Geometry check sheet. Reference: the model listing, model coordinates, mm. A direction names the side the tool comes from. Coordinates: 2 decimals unless noted, no trailing zeros. Write each loop counter-clockwise with the first axis right and the second up, starting at its lowest first coordinate (ties: lowest second). Pieces come first, ordered by that corner, then holes. Notation, with made-up numbers: M -35,3 L 16,3 A34 ccw 16,34 Z; hole C 82.5,70.5 d4. An arc over 180 degrees is marked long. Write each question's results on one line, items separated by ' | '.
```python
from build123d import *

# Parameters (mm, degrees)
REVOLVE1_ANGLE = 72


with BuildPart() as part:
    # Sketch1 → Revolve1 (revolve)
    with BuildSketch(Plane.XY):
        with BuildLine():
            ThreePointArc((-52.157480315, 97.330708661), (-49.814334564, 102.987562911), (-44.157480315, 105.330708661))
            Line((-44.157480315, 105.330708661), (6.842519685, 105.330708661))
            ThreePointArc((6.842519685, 105.330708661), (12.499373935, 102.987562911), (14.842519685, 97.330708661))
            Line((14.842519685, 97.330708661), (14.842519685, 70.330708661))
            Line((14.842519685, 70.330708661), (10.842519685, 70.330708661))
            Line((10.842519685, 70.330708661), (10.842519685, 97.330708661))
            ThreePointArc((10.842519685, 97.330708661), (9.67094681, 100.159135786), (6.842519685, 101.330708661))
            Line((6.842519685, 101.330708661), (-44.157480315, 101.330708661))
            ThreePointArc((-44.157480315, 101.330708661), (-46.98590744, 100.159135786), (-48.157480315, 97.330708661))
            Line((-48.157480315, 97.330708661), (-48.157480315, 70.330708661))
            Line((-48.157480315, 70.330708661), (-52.157480315, 70.330708661))
            Line((-52.157480315, 70.330708661), (-52.157480315, 97.330708661))
        make_face()
    revolve(axis=Axis((14.842519685, -1144.669291339, 0), (-1, 0, 0)), revolution_arc=REVOLVE1_ANGLE)


solid = part.part
```
Q1. Depth check by flat-ended pin: P1, Ø12, axis at x = 7, y = -155.5, coming from the +Z side; P2, Ø8, axis at x = -5, z = -196, coming from the -Y side; P3, Ø6, axis at x = 1.5, z = -266, coming from the +Y side. Enter the tip coordinate at first touch or a pass-through.
Geometry check:
P1: stops at z = -699.02 | P2: stops at y = 85.17 | P3: stops at y = 77.35
Q2. Access from +Z, -Z, +X, -X, +Y, -Y to the whole of each face (thin tool, end or side, straight path). Record for faces 4 (the cylindrical face through (12.815, -155.47, -705.485)), 5 (the cylindrical face through (-19.014, -130.231, -723.485)).
Geometry check:
face 4: +Z, +X, -X, -Y | face 5: +Z, -Y
Q3. Sectioned sample at A-A on x = -7.5. Record the cut outline in (y, z).
Geometry check:
outline: M -759.63,-1185.02 L -758.4,-1188.82 A1250 ccw 105.33,0 L 101.33,0 A1246 cw Z
Q4. Scan lines: probe 1 along Z at (x, y) = (-16.5, -42.5); probe 2 along Z at (x, y) = (-8.5, -371); probe 3 along Y at (x, z) = (-9.5, -945). Record each from-to range of solid material in increasing order.
Geometry check:
probe 1: z = -589.68 to -581.15 | probe 2: z = -981.8 to -976.7 | probe 3: y = -332.58 to -326.45
Q5. Mould release check, pull along X, two halves, no side actions. Record for faces 1 (the flat face through (14.843, -145, -725)), 2 (the flat face through (10.843, -141, -725)), 3 (the flat face through (-16, 102, 0)): pulls with the +X half, pulls with the -X half, needs draft (parallel to the pull), parting line crosses it, or undercut.
Geometry check:
face 1: pulls with the +X half | face 2: undercut | face 3: needs draft
